```python
from build123d import *

# Parameters (mm, degrees)
BOSS_EXTRUDE1_DEPTH = 40
SKETCH2_R           = 18
BOSS_EXTRUDE2_DEPTH = 30.2
SKETCH3_R           = 11
BOSS_EXTRUDE3_DEPTH = 2
SKETCH4_R           = 4
BOSS_EXTRUDE4_DEPTH = 17.25


with BuildPart() as part:
    # Sketch1 → Boss-Extrude1 (new body)
    with BuildSketch(Plane.XY):
        Polygon((-21, 18), (-18, 21), (18, 21), (21, 18), (21, -18), (18, -21), (-18, -21), (-21, -18), align=None)
    extrude(amount=BOSS_EXTRUDE1_DEPTH)

    # Sketch2 → Boss-Extrude2 (add)
    with BuildSketch(Plane.XY.offset(40)):
        Circle(SKETCH2_R)
    extrude(amount=BOSS_EXTRUDE2_DEPTH)

    # Sketch3 → Boss-Extrude3 (add)
    with BuildSketch(Plane.XY.offset(70.2)):
        Circle(SKETCH3_R)
    extrude(amount=BOSS_EXTRUDE3_DEPTH)

    # Sketch4 → Boss-Extrude4 (add)
    with BuildSketch(Plane.XY.offset(72.2)):
        Circle(SKETCH4_R)
    extrude(amount=BOSS_EXTRUDE4_DEPTH)


solid = part.part
```
Part model, mm, in its own coordinate system. A direction names the side the tool comes from. Round coordinates to 2 decimals unless told otherwise and drop trailing zeros. Write each loop counter-clockwise with the first axis right and the second up, starting at its lowest first coordinate (ties: lowest second). Pieces come first, ordered by that corner, then holes. Notation, with made-up numbers: M 84,86.5 L 131,86.5 A18 cw 131,106.5 Z; hole C -29.5,58 d3. An arc over 180 degrees is marked long. Answer as CSV lines item,"result". Start each with the question number.
1) Band-saw the part on A-A (x = 0). List the corners of the cut face in (y, z), then the cut area to 3 significant figures.
2) Which spindle directions (+Z, -Z, +X, -X, +Y, -Y) get a long thin tool onto all of the face, cutting with end or side? Do faces 1 (the face through (-8, -8, 70.2)), 2 (the face through (21, 0, 20)). Say none if no direction does.
3) Band-saw the part on D-D (y = 6.5). List the corners of the cut face in (x, z), then the cut area to 3 significant figures.
4) Drill centre lines: L1, parallel to Z at x = -0.5, y = 15.5; L2, parallel to Z at x = 14.5, y = -14; L3, parallel to Y at x = -15, z = 52. Where is each one in solid material? Low to high.
5) Drop flat-ended pins along their axis: pin 1 (2 mm diameter, centred on x = 11.5, z = 59.5, fed in from -Y); pin 2 (5 mm diameter, centred on x = 14, z = 45.5, fed in from +Y); pin 3 (21 mm diameter, centred on x = -10.5, y = -8.5, fed in from +Z); pin 4 (10 mm diameter, centred on y = 13, z = 69.5, fed in from -X). Give the stop position or say it passes through.
6) Band-saw the part on C-C (z = 74.5). List the corners of the cut face in (x, y), then the cut area to 3 significant figures.
Worked out:
1,outline,"M -21,0 L 21,0 L 21,40 L 18,40 L 18,70.2 L 11,70.2 L 11,72.2 L 4,72.2 L 4,89.45 L -4,89.45 L -4,72.2 L -11,72.2 L -11,70.2 L -18,70.2 L -18,40 L -21,40 Z"
1,area,"2,950 mm²"
2,face 1,"+Z"
2,face 2,"+Z, -Z, +X, +Y, -Y"
3,outline,"M -21,0 L 21,0 L 21,40 L 16.79,40 L 16.79,70.2 L 8.87,70.2 L 8.87,72.2 L -8.87,72.2 L -8.87,70.2 L -16.79,70.2 L -16.79,40 L -21,40 Z"
3,area,"2,730 mm²"
4,L1,"0 to 70.2"
4,L2,"0 to 40"
4,L3,"-9.95 to 9.95"
5,pin 1,"y = -14.62"
5,pin 2,"y = 13.85"
5,pin 3,"z = 89.45"
5,pin 4,"x = -16.12"
6,outline,"C 0,0 d8"
6,area,"50.3 mm²"
